Can you work these out from the model? Positions are in its coordinate system, mm. A direction names the side the tool comes from. Give positions to 0.01 mm unless a question says otherwise; leave off trailing zeros. Write each loop counter-clockwise with the first axis right and the second up, starting at its lowest first coordinate (ties: lowest second). Pieces come first, ordered by that corner, then holes. Notation, with made-up numbers: (-21.5, 81.5) -> (37.5, 81.5) arc R21 ccw to (37.5, 106.5) -> close; hole circle Ø3 at (45, -2). An arc over 180 degrees is marked (long way). Answer as CSV lines item,"result". Start each with the question number.
1. If we section it at B-B on x = 0: Write out the boundary of the cut face in (y, z).
2. I need wall thicknesses on line 1 (Y direction, x = 0, z = 1.3); line 2 (Y direction, x = 14.5, z = 3.55); line 3 (Y direction, x = -14, z = 2.45). Which ranges of each line are inside material? Lowest first, please. Write a range as [from, to].
3. If we mould it in two halves opening along X, with no side actions, what happens to faces 1 (the face through (-23, 16.8, 2)), 2 (the face through (-15.17, -14.91, 0.99)), 3 (the face through (-14.8, 14.8, 2)), 4 (the face through (24.901, 0, 2))? For each: pulls with the +X half, pulls with the -X half, needs draft (parallel to the pull), parting line crosses it, or undercut.
4. I'm going to push flat-ended pins straight in: P1, Ø3, axis at x = -14.5, y = -17, coming from the +Z side; P2, Ø3.5, axis at x = 16.02, y = 16.02, coming from the +Z side; P3, Ø2, axis at x = -16.02, y = -16.02, coming from the -Z side; P4, Ø1.1, axis at x = 23, z = 3, coming from the -Y side. Where does each tip first touch, or does it pass through?
5. If we section it at D-D on z = 1.2: Write out the boundary of the cut face in (x, y), plus the area to 3 significant figures.
6. If we section it at A-A on y = -15.5: Write out the boundary of the cut face in (x, z).
7. On a 3-axis mill with a long thin cutter (end or side, diameter ignored), from which of +Z, -Z, +X, -X, +Y, -Y can I reach the whole of each face in a straight line? I mean faces 5 (the face through (-16.8, 23, 2)), 6 (the face through (16.8, 23, 2)), 7 (the face through (13.294, 16.378, 3.479)), 8 (the face through (23, -16.8, 2)). Say none if no direction works.
Autodesk Inventor part; units mm, degrees
ref_plane "YZ Plane" through (0, 0, 0) normal (1, 0, 0) x (0, 1, 0)
ref_plane "XZ Plane" through (0, 0, 0) normal (0, 1, 0) x (-1, 0, 0)
ref_plane "XY Plane" through (0, 0, 0) normal (0, 0, 1) x (1, 0, 0)
sketch "Sketch1" plane through (0, 0, 0) normal (0, 0, 1) x (1, 0, 0)
  line L0 (-39.3843, 0) -> (62.0012, 0) construction
  line L1 (0, -36.6008) -> (0, 45.3001) construction
  line L2 (0, 0) -> (33.6, 33.6) construction
  line L3 (0, 0) -> (47.5176, 0) construction
  line L4 (0, 24.9006) -> (16.8, 24.9006)
  line L5 (16.8, 24.9006) -> (16.8, 21.2406)
  line L6 (16.8, 21.2406) -> (19.0203, 19.0203)
  line L7 (24.9006, 0) -> (24.9006, 16.8)
  line L8 (24.9006, 16.8) -> (21.2406, 16.8)
  line L9 (21.2406, 16.8) -> (19.0203, 19.0203)
  line L10 (0, 24.9006) -> (-16.8, 24.9006)
  line L11 (-16.8, 24.9006) -> (-16.8, 21.2406)
  line L12 (-16.8, 21.2406) -> (-19.0203, 19.0203)
  line L13 (-24.9006, 0) -> (-24.9006, 16.8)
  line L14 (-24.9006, 16.8) -> (-21.2406, 16.8)
  line L15 (-21.2406, 16.8) -> (-19.0203, 19.0203)
  line L16 (0, -24.9006) -> (16.8, -24.9006)
  line L17 (16.8, -24.9006) -> (16.8, -21.2406)
  line L18 (16.8, -21.2406) -> (19.0203, -19.0203)
  line L19 (24.9006, 0) -> (24.9006, -16.8)
  line L20 (24.9006, -16.8) -> (21.2406, -16.8)
  line L21 (21.2406, -16.8) -> (19.0203, -19.0203)
  line L22 (0, -24.9006) -> (-16.8, -24.9006)
  line L23 (-16.8, -24.9006) -> (-16.8, -21.2406)
  line L24 (-16.8, -21.2406) -> (-19.0203, -19.0203)
  line L25 (-24.9006, 0) -> (-24.9006, -16.8)
  line L26 (-24.9006, -16.8) -> (-21.2406, -16.8)
  line L27 (-21.2406, -16.8) -> (-19.0203, -19.0203)
  circle A0 centre (0, 0) radius 12.5
  dimension "d0" = 45
  dimension "d1" = 16.8
  dimension "d2" = 3.66
  dimension "d3" = 3.14
  dimension "d4" = 25
extrude "Extrusion1" add sketch "Sketch1" along normal blind 5
sketch "Sketch2" plane through (0, 0, 5) normal (0, 0, 1) x (1, 0, 0)
  circle A0 centre (0, 0) radius 12.5 construction
  line L0 (16.8, 24.9006) -> (-16.8, 24.9006) construction
  line L1 (-16.8, 24.9006) -> (-16.8, 21.2406) construction
  line L2 (-16.8, 21.2406) -> (-21.2406, 16.8) construction
  line L3 (-21.2406, 16.8) -> (-24.9006, 16.8) construction
  line L4 (-24.9006, 16.8) -> (-24.9006, -16.8) construction
  line L5 (-24.9006, -16.8) -> (-21.2406, -16.8) construction
  line L6 (-21.2406, -16.8) -> (-16.8, -21.2406) construction
  line L7 (-16.8, -21.2406) -> (-16.8, -24.9006) construction
  line L8 (-16.8, -24.9006) -> (16.8, -24.9006) construction
  line L9 (16.8, -24.9006) -> (16.8, -21.2406) construction
  line L10 (16.8, -21.2406) -> (21.2406, -16.8) construction
  line L11 (21.2406, -16.8) -> (24.9006, -16.8) construction
  line L12 (24.9006, -16.8) -> (24.9006, 16.8) construction
  line L13 (24.9006, 16.8) -> (21.2406, 16.8) construction
  line L14 (21.2406, 16.8) -> (16.8, 21.2406) construction
  line L15 (16.8, 21.2406) -> (16.8, 24.9006) construction
  circle A1 centre (16.0203, -16.0203) radius 2.1846 construction
  circle A2 centre (-16.0203, -16.0203) radius 2.1846 construction
  circle A3 centre (-16.0203, 16.0203) radius 2.1846 construction
  circle A4 centre (16.0203, 16.0203) radius 2.1846 construction
  circle A5 centre (0, 0) radius 14 construction
  line L16 (-19.0203, 17.0203) -> (-19.0203, -17.0203) construction
  arc A6 (-17.0203, 19.0203) -> (-19.0203, 17.0203) centre (-17.0203, 17.0203) ccw construction
  line L17 (17.0203, 19.0203) -> (-17.0203, 19.0203) construction
  arc A7 (19.0203, 17.0203) -> (17.0203, 19.0203) centre (17.0203, 17.0203) ccw construction
  line L18 (19.0203, -17.0203) -> (19.0203, 17.0203) construction
  arc A8 (17.0203, -19.0203) -> (19.0203, -17.0203) centre (17.0203, -17.0203) ccw construction
  line L19 (-17.0203, -19.0203) -> (17.0203, -19.0203) construction
  arc A9 (-19.0203, -17.0203) -> (-17.0203, -19.0203) centre (-17.0203, -17.0203) ccw construction
hole "Hole1" at (-16.0203, 16.0203, 5) at (16.0203, 16.0203, 5) at (16.0203, -16.0203, 5) at (-16.0203, -16.0203, 5) direction (0, 0, -1) diameter 2.8 end through all counterbore diameter 5.5 counterbore depth 3
properties part number "20_Cube_insert_Sample_holder_magnetic"
Computed values:
1,outline,"(-24.9, 0) -> (-12.5, 0) -> (-12.5, 5) -> (-24.9, 5) -> close; (12.5, 0) -> (24.9, 0) -> (24.9, 5) -> (12.5, 5) -> close"
2,line 1,"y = [-24.9, -12.5], [12.5, 24.9]"
2,line 2,"y = [-24.9, -18.31], [-13.73, 13.73], [18.31, 24.9]"
2,line 3,"y = [-24.9, -17.89], [-14.15, 14.15], [17.89, 24.9]"
3,face 1,"needs draft"
3,face 2,"undercut"
3,face 3,"undercut"
3,face 4,"pulls with the +X half"
4,P1,"stops at z = 5"
4,P2,"stops at z = 2"
4,P3,"passes through"
4,P4,"stops at y = -16.8"
5,outline,"(-24.9, -16.8) -> (-21.24, -16.8) -> (-16.8, -21.24) -> (-16.8, -24.9) -> (16.8, -24.9) -> (16.8, -21.24) -> (21.24, -16.8) -> (24.9, -16.8) -> (24.9, 16.8) -> (21.24, 16.8) -> (16.8, 21.24) -> (16.8, 24.9) -> (-16.8, 24.9) -> (-16.8, 21.24) -> (-21.24, 16.8) -> (-24.9, 16.8) -> close; hole circle Ø2.8 at (-16.02, -16.02); hole circle Ø2.8 at (-16.02, 16.02); hole circle Ø25 at (0, 0); hole circle Ø2.8 at (16.02, -16.02); hole circle Ø2.8 at (16.02, 16.02)"
5,area,"1,740 mm2"
6,outline,"(-24.9, 0) -> (-17.32, 0) -> (-17.32, 2) -> (-18.72, 2) -> (-18.72, 5) -> (-24.9, 5) -> close; (-14.72, 0) -> (14.72, 0) -> (14.72, 2) -> (13.32, 2) -> (13.32, 5) -> (-13.32, 5) -> (-13.32, 2) -> (-14.72, 2) -> close; (17.32, 0) -> (24.9, 0) -> (24.9, 5) -> (18.72, 5) -> (18.72, 2) -> (17.32, 2) -> close"
7,face 5,"+Z, -Z, -X, +Y"
7,face 6,"+Z, -Z, +X, +Y"
7,face 7,"+Z"
7,face 8,"+Z, -Z, +X, -Y"
